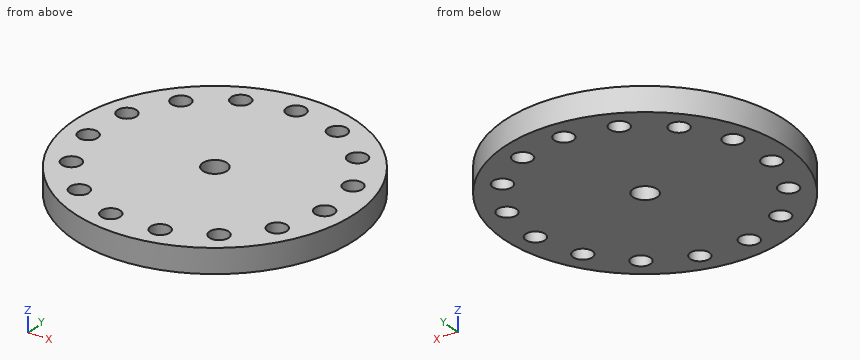
Autodesk Inventor part; units mm, degrees
ref_plane "YZ Plane" through (0, 0, 0) normal (1, 0, 0) x (0, 1, 0)
ref_plane "XZ Plane" through (0, 0, 0) normal (0, 1, 0) x (-1, 0, 0)
ref_plane "XY Plane" through (0, 0, 0) normal (0, 0, 1) x (1, 0, 0)
sketch "Skizze3" plane through (0, 0, 0) normal (0, 0, 1) x (1, 0, 0)
  circle A0 centre (0, 0) radius 11
  line L0 (-11, 11) -> (11, 11)
  line L1 (11, 11) -> (11, -11)
  line L2 (11, -11) -> (-11, -11)
  line L3 (-11, -11) -> (-11, 11)
  dimension "d13" = 22
extrude "Extrusion3" add sketch "Skizze3" along normal blind 1.9 contours A0
sketch "Skizze4" plane through (0, 0, 1.9) normal (0, 0, 1) x (1, 0, 0)
  circle A0 centre (0, 0) radius 11
  circle A1 centre (0, 9.2) radius 0.75
  line L0 (0, 9.2) -> (0, 11)
  dimension "d17" = 1.5
  dimension "d26" = 1.8
extrude "Extrusion4" cut sketch "Skizze4" against normal through all contours A1
pattern_circular "Runde Anordnung1" count 15 over 360 about axis through (0, 0, -10) along (0, 0, 1) of "Extrusion4"
sketch "Skizze5" plane through (0, 0, 1.9) normal (0, 0, 1) x (1, 0, 0)
  circle A0 centre (0, 0) radius 11
  circle A1 centre (0, 0) radius 0.95
  dimension "d23" = 1.9
extrude "Extrusion5" cut sketch "Skizze5" against normal through all contours A1
properties part number "EncoderWheel2"
The listing builds one solid part. Answer for the finished solid, in the listing's coordinates (mm). Round coordinates to 2 decimals unless told otherwise and drop trailing zeros. Loops run counter-clockwise (first coordinate to the right, second up) from the corner with the lowest first, then second, coordinate; pieces in that order, holes last. Notation, with made-up numbers: (28.5, 53.25) - (50.5, 53.25) arc R15 cw to (50.5, 76.25) - close; hole circle Ø1 at (5, 22.5). An arc over 180 degrees is marked (long way). Return JSON: item names as keys, results as strings. Group by question number.
1. The part is cut by section D-D on y = 4. Determine the outline of the cut face in (x, z).
2. The part is cut by section B-B on x = 3.75. Determine the outline of the cut face in (y, z), then the cut area to 3 significant figures.
3. Consider probe 1 along X at (y, z) = (-9.25, 0.2); probe 2 along X at (y, z) = (5.75, 1.35); probe 3 along Y at (x, z) = (0.5, 0.85). Determine where each line is inside the solid, lowest interval first.
4. Each of these flat-tipped pins is pushed along its axis until it touches: P1, Ø2, axis at x = -1.91, y = -9, coming from the +Z side; P2, Ø1.4, axis at x = -5.41, y = -7.44, coming from the +Z side. Where does it stop, or does it pass through?
5. The part is cut by section A-A on x = 0. Determine the outline of the cut face in (y, z), then the cut area to 3 significant figures.
Resolved:
{
 "1": {"outline": "(-10.25, 0) - (10.25, 0) - (10.25, 1.9) - (-10.25, 1.9) - close"},
 "2": {"outline": "(-10.34, 0) - (7.65, 0) - (7.65, 1.9) - (-10.34, 1.9) - close; (9.15, 0) - (10.34, 0) - (10.34, 1.9) - (9.15, 1.9) - close", "area": "36.4 mm²"},
 "3": {"probe 1": "x = -5.95 to -2.62, -1.21 to 1.21, 2.62 to 5.95", "probe 2": "x = -9.38 to -7.47, -6.21 to 6.21, 7.47 to 9.38", "probe 3": "y = -10.99 to -0.81, 0.81 to 8.64, 9.76 to 10.99"},
 "4": {"P1": "stops at z = 1.9", "P2": "passes through"},
 "5": {"outline": "(-11, 0) - (-0.95, 0) - (-0.95, 1.9) - (-11, 1.9) - close; (0.95, 0) - (8.45, 0) - (8.45, 1.9) - (0.95, 1.9) - close; (9.95, 0) - (11, 0) - (11, 1.9) - (9.95, 1.9) - close", "area": "35.3 mm²"}
}
